from build123d import *

# Parameters (mm, degrees)
ESBO_O1_W                = 113
ESBO_O1_H                = 25
RESSALTO_EXTRUS_O1_DEPTH = 5
CORTE_EXTRUS_O1_DEPTH    = 5
ESBO_O4_R                = 1
ESBO_O4_R_2              = 1.1
CORTE_EXTRUS_O2_DEPTH    = 76
ESBO_O5_R                = 2
CORTE_EXTRUS_O3_DEPTH    = 10
ESBO_O6_W                = 30
ESBO_O6_H                = 6
CORTE_EXTRUS_O4_DEPTH    = 10


with BuildPart() as part:
    # Esboço1 → Ressalto-extrusão1 (new body)
    with BuildSketch(Plane(origin=(0, 0, 0), x_dir=(1, 0, 0), z_dir=(0, 1, 0))):
        with Locations((9.231716451, 5.983979594)):
            Rectangle(ESBO_O1_W, ESBO_O1_H)
    extrude(amount=RESSALTO_EXTRUS_O1_DEPTH)

    # Esboço2 → Corte-extrusão1 (cut)
    with BuildSketch(Plane(origin=(0, 5, 0), x_dir=(1, 0, 0), z_dir=(0, 1, 0))):
        Polygon((65.731716451, 0.283979594), (62.231716451, 0.283979594), (62.231716451, -1.516020406), (60.731716451, -1.516020406), (60.731716451, 0.283979594), (58.731716451, 0.283979594), (58.731716451, 2.283979594), (60.731716451, 2.283979594), (60.731716451, 4.083979594), (62.231716451, 4.083979594), (62.231716451, 2.283979594), (65.731716451, 2.283979594), align=None)
        Polygon((65.731716451, 9.683979594), (62.231716451, 9.683979594), (62.231716451, 7.883979594), (60.731716451, 7.883979594), (60.731716451, 9.683979594), (58.731716451, 9.683979594), (58.731716451, 11.683979594), (60.731716451, 11.683979594), (60.731716451, 13.483979594), (62.231716451, 13.483979594), (62.231716451, 11.683979594), (65.731716451, 11.683979594), align=None)
    corte_extrus_o1 = extrude(amount=-CORTE_EXTRUS_O1_DEPTH, mode=Mode.SUBTRACT)

    # Esboço4 → Corte-extrusão2 (cut)
    with BuildSketch(Plane(origin=(0, 5, 0), x_dir=(1, 0, 0), z_dir=(0, 1, 0))):
        with Locations(Location((-25.688283549, 12.683979594, 0), (0, 0, 270))):
            Circle(ESBO_O4_R)
        with Locations(Location((44.151716451, 12.683979594, 0), (0, 0, 270))):
            Circle(ESBO_O4_R_2)
    extrude(amount=-CORTE_EXTRUS_O2_DEPTH, mode=Mode.SUBTRACT)

    # Esboço5 → Corte-extrusão3 (cut)
    with BuildSketch(Plane(origin=(0, 5, 0), x_dir=(1, 0, 0), z_dir=(0, 1, 0))):
        with Locations(Location((-34.268283549, 13.483979594, 0), (0, 0, 270))):
            Circle(ESBO_O5_R)
        with Locations(Location((-34.268283549, -1.516020406, 0), (0, 0, 270))):
            Circle(ESBO_O5_R)
        with Locations(Location((52.731716451, 13.483979594, 0), (0, 0, 270))):
            Circle(ESBO_O5_R)
        with Locations(Location((52.731716451, -1.516020406, 0), (0, 0, 270))):
            Circle(ESBO_O5_R)
    extrude(amount=-CORTE_EXTRUS_O3_DEPTH, mode=Mode.SUBTRACT)

    # Esboço6 → Corte-extrusão4 (cut)
    with BuildSketch(Plane(origin=(0, 5, 0), x_dir=(1, 0, 0), z_dir=(0, 1, 0))):
        with Locations((24.231716451, 10.483979594)):
            Rectangle(ESBO_O6_W, ESBO_O6_H)
    corte_extrus_o4 = extrude(amount=-CORTE_EXTRUS_O4_DEPTH, mode=Mode.SUBTRACT)

    # Espelhar1: Corte-extrusão1, Corte-extrusão4 across plane
    add(corte_extrus_o1.mirror(Plane(origin=(9.231716451, 0, 0), x_dir=(0, 0, 1), z_dir=(1, 0, 0))), mode=Mode.SUBTRACT)
    add(corte_extrus_o4.mirror(Plane(origin=(9.231716451, 0, 0), x_dir=(0, 0, 1), z_dir=(1, 0, 0))), mode=Mode.SUBTRACT)


solid = part.part
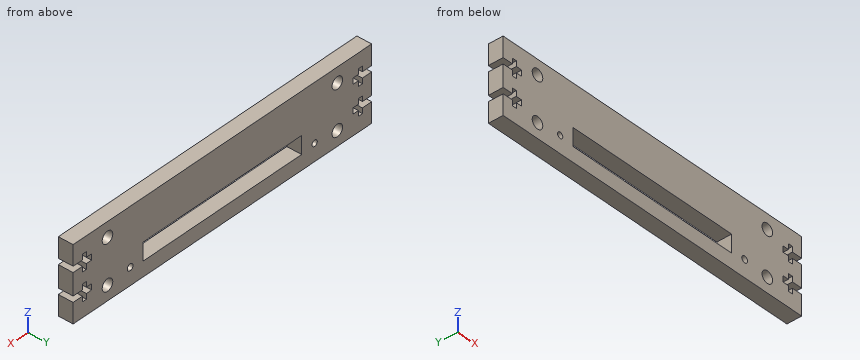
The listing builds one solid part. Answer for the finished solid, in the listing's coordinates (mm). Give positions to 0.01 mm unless a question says otherwise; leave off trailing zeros. Write each loop counter-clockwise with the first axis right and the second up, starting at its lowest first coordinate (ties: lowest second). Pieces come first, ordered by that corner, then holes. Notation, with made-up numbers: (83, -30) -> (106, -30) arc R9 cw to (106, -23) -> close; hole circle Ø8 at (61.5, 68.5). An arc over 180 degrees is marked (long way). Use a Markdown table: item, result.
(1) Section B-B, the plane y = 2.05 is taken. Give the number of separate pieces and of enclosed holes in the cut face, then the cut area to 3 significant figures.
Return value:
| item | result |
|---|---|
| separate pieces | 1 |
| enclosed holes | 7 |
| area | 2,330 mm2 |
(2) Section A-A, the plane x = 28 is taken. Determine the outline of the cut face in (y, z).
Return value:
| item | result |
|---|---|
| outline | (0, -18.48) -> (5, -18.48) -> (5, -13.48) -> (0, -13.48) -> close; (0, -7.48) -> (5, -7.48) -> (5, 6.52) -> (0, 6.52) -> close |
(3) Find the intervals of material crossed by probe 1 along Z at (x, y) = (52.5, 1.2); probe 2 along X at (y, z) = (4.7, -2.75); probe 3 along Z at (x, y) = (-11.5, 4.3), in increasing order. Write a range as from..to.
Return value:
| item | result |
|---|---|
| probe 1 | -18.48..-15.47, -11.5..-0.47, 3.5..6.52 |
| probe 2 | -47.27..-43.77, -42.27..60.73, 62.23..65.73 |
| probe 3 | -18.48..-13.48, -7.48..6.52 |
(4) A flat-ended cylindrical pin translates along its axis: P1, Ø0.6, axis at y = 3.5, z = -1, coming from the +X side. Find the tip coordinate at first contact, or state that the pin passes through.
Return value:
| item | result |
|---|---|
| P1 | x = 58.73 |
